```python
from build123d import *

# Parameters (mm, degrees)
F1_DEPTH = 25
F2_R     = 1


# Not quite as in the source:
# - a feature names something its author has since deleted; it is built from what else it names


with BuildPart() as f1:
    # F0 (on Top) → F1 (new body)
    with BuildSketch(Plane.XY):
        Polygon((0, -2), (0, 0), (-37.5, 0), (-37.5, 8.1967763358), (-56.72952592, 5.6744525365), (-33.382604787, -17.6724685966), (-11, -2), align=None)
        Polygon((-39.5, -2), (-14.4868935912, -2), (-33.1550573032, -15.0715889556), (-52.4458532095, 4.2192069507), (-39.5, 5.9173056865), align=None, mode=Mode.SUBTRACT)
        Polygon((37.5, 0), (0, 0), (0, -2), (11, -2), (33.382604787, -17.6724685966), (56.72952592, 5.6744525365), (37.5, 8.1967763358), align=None)
        Polygon((33.1550573032, -15.0715889556), (14.4868935912, -2), (39.5, -2), (39.5, 5.9173056865), (52.4458532095, 4.2192069507), align=None, mode=Mode.SUBTRACT)
    extrude(amount=F1_DEPTH)

    # F2
    f2_edges = [f1.edges().sort_by_distance(p)[0] for p in [
        (-37.5, 8.196776, 12.5),
        (-56.729526, 5.674453, 12.5),
        (-33.382605, -17.672469, 12.5),
        (-37.5, 0, 12.5),
        (-39.5, -2, 12.5),
        (37.5, 0, 12.5),
        (37.5, 8.196776, 12.5),
        (56.729526, 5.674453, 12.5),
        (39.5, -2, 12.5),
        (33.382605, -17.672469, 12.5),
        (14.486894, -2, 12.5),
        (-14.486894, -2, 12.5),
        (-39.5, 5.917306, 12.5),
        (-33.155057, -15.071589, 12.5),
        (39.5, 5.917306, 12.5),
        (33.155057, -15.071589, 12.5),
    ]]
    fillet(f2_edges, radius=F2_R)


solid = f1.part
```
Could you check a few things on this model? Use its own coordinates, in mm. A direction names the side the tool comes from. Coordinates: 2 decimals unless noted, no trailing zeros. Order: outer loops, then holes, each group sorted by start corner. A loop starts at its lowest first (then second) coordinate and runs counter-clockwise, first axis right, second up. Notation, with made-up numbers: M -26,38 L 7,38 A17 cw 7,45 Z; hole C -15,48.5 d8. An arc over 180 degrees is marked long. Use one line per item in the form item = value. Start each with the question number.
1. On a 3-axis mill with a long thin cutter (end or side, diameter ignored), from which of +Z, -Z, +X, -X, +Y, -Y can I reach the whole of each face in a straight line? I mean faces 1 (the flat face through (21.7, -9.49, 12.32)), 2 (the flat face through (44.486, -6.569, 12.325)), 3 (the flat face through (46.79, 6.98, 12.32)), 4 (the cylindrical face through (-16.71, -2.68, 12.68)), 5 (the flat face through (-37.5, 4, 12)). Say none if no direction works.
2. Suppose I cut it at A-A on y = 2.5. Write out the boundary of the cut face in (x, z), then the cut area to 3 significant figures.
3. Please list where these lines run through material, in increasing order: line 1 (X direction, y = -9.25, z = 7.75); line 2 (X direction, y = 3.75, z = 24.25); line 3 (Y direction, x = 47, z = 5).
4. Suppose I cut it at B-B on z = 1.5. Count the separate pieces of the cut face and the enclosed holes in it, then the cut area to 3 significant figures.
5. Suppose I cut it at D-D on y = -11.5. Write out the boundary of the cut face in (x, z), then the cut area to 3 significant figures.
6. For pin 1 (6 mm diameter, centred on x = -13, z = 19, fed in from -Y); pin 2 (12 mm diameter, centred on y = -7.5, z = 19, fed in from +X); pin 3 (3 mm diameter, centred on y = 1, z = 10.5, fed in from -X), each with a flat end and sliding along its axis, tell me the tip position at first contact or that it passes through.
7. We'd pull the mould along X, two halves only. Please class faces 6 (the flat face through (-44.785, -6.27, 12.325)), 7 (the flat face through (-0.3, -1.8, 25)), 8 (the flat face through (-28, -2, 12)): +X half, -X half, draft (parallel to the pull), parting line (faces both ways), or undercut.
8. Suppose I cut it at C-C on x = -26.5. Write out the boundary of the cut face in (y, z), then the cut area to 3 significant figures.
Geometry says:
q1.face_1 = +Z, -Z, -Y
q1.face_2 = +Z, -Z, +X, -Y
q1.face_3 = +Z, -Z, +X, +Y
q1.face_4 = +Z, -Z
q1.face_5 = +Z, -Z, +Y
q2.outline = M -53.56,0 L -50.73,0 L -50.73,25 L -53.56,25 Z; M -39.5,0 L -37.5,0 L -37.5,25 L -39.5,25 Z; M 37.5,0 L 39.5,0 L 39.5,25 L 37.5,25 Z; M 50.73,0 L 53.56,0 L 53.56,25 L 50.73,25 Z
q2.area = 241 mm^2
q3.line_1 = -41.81 to -38.98, -24.84 to -21.35, 21.35 to 24.84, 38.98 to 41.81
q3.line_2 = -54.81 to -51.98, -39.5 to -37.5, 37.5 to 39.5, 51.98 to 54.81
q3.line_3 = -4.06 to -1.23, 4.93 to 6.95
q4.separate_pieces = 1
q4.enclosed_holes = 2
q4.area = 474 mm^2
q5.outline = M -39.56,0 L -36.73,0 L -36.73,25 L -39.56,25 Z; M -28.05,0 L -24.57,0 L -24.57,25 L -28.05,25 Z; M 24.57,0 L 28.05,0 L 28.05,25 L 24.57,25 Z; M 36.73,0 L 39.56,0 L 39.56,25 L 36.73,25 Z
q5.area = 316 mm^2
q6.pin_1 = -5.5
q6.pin_2 = 49.56
q6.pin_3 = -53.56
q7.face_6 = -X half
q7.face_7 = draft
q7.face_8 = undercut
q8.outline = M -12.85,0 L -10.41,0 L -10.41,25 L -12.85,25 Z; M -2,0 L 0,0 L 0,25 L -2,25 Z
q8.area = 111 mm^2
